```python
from build123d import *

# Parameters (mm, degrees)
F1_DEPTH  = 63.5
F2_R      = 12.7
F3_W      = 38.1
F3_H      = 6.35
F4_DEPTH  = 25.4
F5_W      = 31.75
F5_H      = 7.874
F6_DEPTH  = 25.4
F8_R      = 15.103409
F9_DEPTH  = 4.572
F10_R     = 7.112
F11_DEPTH = 27.179
F12_DEPTH = 25.4
F13_DEPTH = 12.701


with BuildPart() as f1:
    # F0 (on Front) → F1 (new body)
    with BuildSketch(Plane.XZ):
        Polygon((0, 47.752), (0, 0), (60.198, 0), (60.198, -5.08), (63.5, -5.08), (63.5, -19.05), (76.2, -19.05), (76.2, 12.7), (12.7, 12.7), (12.7, 47.752), align=None)
    extrude(amount=F1_DEPTH)

    # F2
    f2_edges = [f1.edges().sort_by_distance(p)[0] for p in [
        (6.35, -63.5, 47.752),
        (6.35, 0, 47.752),
    ]]
    fillet(f2_edges, radius=F2_R)

    # F3 (on face) → F4 (cut)
    with BuildSketch(Plane.YZ.offset(76.2)):
        with Locations((-31.75, -15.875)):
            Rectangle(F3_W, F3_H)
    extrude(amount=-F4_DEPTH, mode=Mode.SUBTRACT)

    # F5 (on face) → F6 (cut)
    with BuildSketch(Plane.XY.offset(12.7)):
        with Locations((44.323, -59.563)):
            Rectangle(F5_W, F5_H)
        with Locations((44.323, -3.937)):
            Rectangle(F5_W, F5_H)
    extrude(amount=-F6_DEPTH, mode=Mode.SUBTRACT)

    # F8 (on face) → F9 (cut)
    with BuildSketch(Plane.XY.offset(12.7)):
        with Locations((45.094591, -31.75)):
            Circle(F8_R)
    extrude(amount=-F9_DEPTH, mode=Mode.SUBTRACT)

    # F10 (on face) → F11 (cut, through all)
    with BuildSketch(Plane.XY.offset(8.128)):
        with Locations((45.094591, -31.75)):
            Circle(F10_R)
    extrude(amount=-F11_DEPTH, mode=Mode.SUBTRACT)

    # F7 (on face) → F12 (cut)
    with BuildSketch(Plane.YZ.offset(12.7)):
        with BuildLine():
            Line((-12.7, 42.926), (-50.8, 42.926))
            ThreePointArc((-50.8, 42.926), (-58.674, 35.052), (-50.8, 27.178))
            Line((-50.8, 27.178), (-12.7, 27.178))
            ThreePointArc((-12.7, 27.178), (-4.826, 35.052), (-12.7, 42.926))
        make_face()
    extrude(amount=-F12_DEPTH, mode=Mode.SUBTRACT)

    # F7 (on face) → F13 (cut, through all)
    with BuildSketch(Plane.YZ.offset(12.7)):
        with BuildLine():
            Line((-12.7, 42.926), (-50.8, 42.926))
            ThreePointArc((-50.8, 42.926), (-58.674, 35.052), (-50.8, 27.178))
            Line((-50.8, 27.178), (-12.7, 27.178))
            ThreePointArc((-12.7, 27.178), (-4.826, 35.052), (-12.7, 42.926))
        make_face()
    extrude(amount=-F13_DEPTH, mode=Mode.SUBTRACT)


solid = f1.part
```
Verification items for the finished model (mm, model axes). A direction names the side the tool comes from. Give positions to 0.01 mm unless a question says otherwise; leave off trailing zeros. Order: outer loops, then holes, each group sorted by start corner. A loop starts at its lowest first (then second) coordinate and runs counter-clockwise, first axis right, second up. Notation, with made-up numbers: (60.5, 61.25) -> (94.5, 61.25) arc R17 ccw to (94.5, 91.25) -> close; hole circle Ø4 at (65.5, 20). An arc over 180 degrees is marked (long way). One line per item, written item: value.
(1) Tool access check on faces 1 (the face through (52, -35, 8.128)), 2 (the face through (6.439, -4.828, 34.879)), 3 (the face through (28.448, -60, 6)). Record the directions out of +Z, -Z, +X, -X, +Y, -Y that give a thin tool (end or side, any length) a straight path to the whole face; none if there is none.
Final values:
face 1: +Z
face 2: +X, -X
face 3: +Z, -Z, -Y
(2) Draft check along X on faces 4 (the face through (6.44, -58.67, 35.23)), 5 (the face through (0, -31, 19)), 6 (the face through (60.198, -31, -2)), 7 (the face through (59.5, -27.21, 10.45)). Enter one of: pulls with the +X half, pulls with the -X half, needs draft (parallel to the pull), parting line crosses it, or undercut.
Final values:
face 4: needs draft
face 5: pulls with the -X half
face 6: undercut
face 7: undercut
(3) Sectioned sample at A-A on y = -31.75. Record the cut outline in (x, z).
Final values:
outline: (0, 0) -> (37.98, 0) -> (37.98, 8.13) -> (29.99, 8.13) -> (29.99, 12.7) -> (12.7, 12.7) -> (12.7, 27.18) -> (0, 27.18) -> close; (0, 42.93) -> (12.7, 42.93) -> (12.7, 47.75) -> (0, 47.75) -> close; (52.21, 0) -> (60.2, 0) -> (60.2, -5.08) -> (63.5, -5.08) -> (63.5, -12.7) -> (76.2, -12.7) -> (76.2, 12.7) -> (60.2, 12.7) -> (60.2, 8.13) -> (52.21, 8.13) -> close
(4) Sectioned sample at B-B on z = -14. Record the cut outline in (x, y).
Final values:
outline: (63.5, -63.5) -> (76.2, -63.5) -> (76.2, -50.8) -> (63.5, -50.8) -> close; (63.5, -12.7) -> (76.2, -12.7) -> (76.2, 0) -> (63.5, 0) -> close
(5) Sectioned sample at C-C on x = 71. Record the cut outline in (y, z).
Final values:
outline: (-63.5, -19.05) -> (-50.8, -19.05) -> (-50.8, -12.7) -> (-12.7, -12.7) -> (-12.7, -19.05) -> (0, -19.05) -> (0, 12.7) -> (-63.5, 12.7) -> close
(6) Gauge pin test, flat ends, axial feed: pin 1 (14 mm diameter, centred on x = 46.5, z = 3.5, fed in from -Y); pin 2 (14 mm diameter, centred on x = 8, y = -40, fed in from -Z); pin 3 (4 mm diameter, centred on x = 40.5, z = 3.5, fed in from +Y); pin 4 (7 mm diameter, centred on x = 71, z = -15.5, fed in from +Y). Record the tip position at first contact, or that the pin passes through.
Final values:
pin 1: y = -55.63
pin 2: z = 0
pin 3: y = -7.87
pin 4: y = 0
(7) Scan lines: line 1 along Z through (x, y) = (8.5, -47); line 2 along X through (y, z) = (-56, 14.5). Record each from-to range of solid material in increasing order. Write a range as [from, to].
Final values:
line 1: [0, 27.18], [42.93, 47.75]
line 2: [0, 12.7]
(8) Sectioned sample at D-D on y = -42.5. Record the cut outline in (x, z), then the cut area to 3 significant figures.
Final values:
outline: (0, 0) -> (60.2, 0) -> (60.2, -5.08) -> (63.5, -5.08) -> (63.5, -12.7) -> (76.2, -12.7) -> (76.2, 12.7) -> (55.7, 12.7) -> (55.7, 8.13) -> (34.49, 8.13) -> (34.49, 12.7) -> (12.7, 12.7) -> (12.7, 27.18) -> (0, 27.18) -> close; (0, 42.93) -> (12.7, 42.93) -> (12.7, 47.75) -> (0, 47.75) -> close
area: 1,290 mm^2
